Input: part model. Units: mm. Frame: model coordinates. A direction names the side the tool comes from. Give positions to 0.01 mm unless a question says otherwise; leave off trailing zeros. Loops run counter-clockwise (first coordinate to the right, second up) from the corner with the lowest first, then second, coordinate; pieces in that order, holes last. Notation, with made-up numbers: (61.5, 19.25) - (93.5, 19.25) arc R15 ccw to (93.5, 42.25) - close; hole circle Ø1 at (-32.75, 0). An arc over 180 degrees is marked (long way). Answer as a JSON object with one key per item and string values. Group by question number.
(1) Pin query (flat end, axial travel): P1, Ø8, axis at x = 6.5, y = 5.5, coming from the -Z side; P2, Ø0.8, axis at y = 13.5, z = 2.5, coming from the -X side; P3, Ø0.8, axis at x = 9.5, z = 2, coming from the -Y side; P4, Ø1.2, axis at y = 13.5, z = 2.5, coming from the +X side. Return the tip coordinate at first contact, or that it passes through.
(2) Section query D-D (z = 0.8). Count the separate pieces of the cut face and the enclosed holes in it, plus the area to 3 significant figures.
(3) Section query A-A (x = 2.5). Return loops of the section in (y, z).
(4) Material intervals for L1, parallel to X at y = 9, z = 2.1; L2, parallel to Z at x = 4.5, y = 6; L3, parallel to Y at x = 2.5, z = 0.55, sorted ascending.
(5) Access query for faces 1 (the flat face through (10, 9.7, 2)), 2 (the flat face through (8.9, 13, 2)), 3 (the flat face through (8.4, 8, 2)), 4 (the flat face through (11.9, 13, 2)). Directions: +Z, -Z, +X, -X, +Y, -Y. A direction counts if a zero-diameter tool reaches every point of the face in a straight line with its end or side. Return the directions, or none.
(6) Section query B-B (y = 13.2). Return loops of the section in (x, z), plus the area to 3 significant figures.
(7) Mould query, pull axis Y, two halves, no side actions, for faces 5 (the flat face through (3.25, 8, 2)), 6 (the flat face through (10, 14.1, 2)), 7 (the flat face through (10, 12.3, 2)). Classes: +Y half, -Y half, draft (parallel to the pull), parting line (faces both ways), or undercut.
(8) Section query C-C (z = 2.55). Return loops of the section in (x, y).
Autodesk Inventor part; units mm, degrees
ref_plane "YZ Plane" through (0, 0, 0) normal (1, 0, 0) x (0, 1, 0)
ref_plane "XZ Plane" through (0, 0, 0) normal (0, 1, 0) x (-1, 0, 0)
ref_plane "XY Plane" through (0, 0, 0) normal (0, 0, 1) x (1, 0, 0)
sketch "Skizze1" plane through (0, 0, 0) normal (0, 0, 1) x (1, 0, 0)
  line L0 (0, 0) -> (20.8, 0)
  line L1 (20.8, 0) -> (20.8, 15.7)
  line L2 (20.8, 15.7) -> (0, 15.7)
  line L3 (0, 15.7) -> (0, 0)
  circle A0 centre (2.5, 13.2) radius 1.55
  circle A1 centre (18.3, 13.2) radius 1.55
  dimension "d0" = 20.8
  dimension "d1" = 15.7
  dimension "d2" = 2.5
  dimension "d3" = 2.5
  dimension "d4" = 2.5
  dimension "d5" = 2.5
  dimension "d6" = 3.1
  dimension "d7" = 3.1
extrude "Grundkörper" add sketch "Skizze1" along normal blind 1.4
sketch "Skizze2" plane through (0, 0, 1.4) normal (0, 0, 1) x (1, 0, 0)
  line L0 (8.4, 5.7) -> (12.4, 5.7)
  line L1 (12.4, 5.7) -> (12.4, 9.7)
  line L2 (12.4, 9.7) -> (8.4, 9.7)
  line L3 (8.4, 9.7) -> (8.4, 5.7)
  line L4 (20.8, 0) -> (20.8, 15.7)
  line L5 (20.8, 15.7) -> (0, 15.7)
  line L6 (1.75, 6.2) -> (3.25, 6.2)
  line L7 (3.25, 6.2) -> (3.25, 9.2)
  line L8 (3.25, 9.2) -> (1.75, 9.2)
  line L9 (1.75, 9.2) -> (1.75, 6.2)
  line L10 (12.4, 7.7) -> (8.4, 7.7) construction
  line L11 (3.25, 7.7) -> (1.75, 7.7) construction
  line L12 (0, 15.7) -> (0, 0) construction
  line L13 (8.9, 14.1) -> (11.9, 14.1)
  line L14 (11.9, 14.1) -> (11.9, 12.3)
  line L15 (11.9, 12.3) -> (8.9, 12.3)
  line L16 (8.9, 12.3) -> (8.9, 14.1)
  line L17 (10.4, 15.7) -> (10.4, 0) construction
  line L18 (0, 0) -> (20.8, 0) construction
  line L19 (10.4, 9.7) -> (10.4, 5.7) construction
  circle A0 centre (2.5, 13.2) radius 1.55 construction
  circle A1 centre (18.3, 13.2) radius 1.55 construction
  line L20 (2.5, 13.2) -> (18.3, 13.2) construction
  line L21 (10.4, 14.1) -> (10.4, 12.3) construction
  line L22 (8.9, 13.2) -> (11.9, 13.2) construction
  line L23 (2.5, 13.2) -> (2.5, 11.65) construction
  line L24 (2.5, 9.2) -> (2.5, 6.2) construction
  dimension "d10" = 4
  dimension "d11" = 4
  dimension "d13" = 6
  dimension "d14" = 3
  dimension "d15" = 1.5
  dimension "d17" = 1.8
  dimension "d18" = 3
extrude "SMDs" add sketch "Skizze2" along normal blind 1.5
sketch "Skizze3" plane through (0, 0, 1.4) normal (0, 0, 1) x (1, 0, 0)
  line L0 (20.8, 15.7) -> (0, 15.7) construction
  line L1 (10.4, 15.7) -> (10.4, 0) construction
  line L2 (0, 0) -> (20.8, 0) construction
  line L3 (0, 15.7) -> (0, 0) construction
  line L4 (0, 1.6) -> (20.8, 1.6) construction
  line L5 (20.8, 0) -> (20.8, 15.7) construction
  point P0 (19.225, 1.6132)
  point P1 (16.685, 1.6132)
  point P2 (14.145, 1.6132)
  point P3 (11.605, 1.6132)
  point P4 (9.065, 1.6132)
  point P5 (6.525, 1.6132)
  point P6 (3.985, 1.6132)
  point P7 (1.445, 1.6132)
  dimension "d28" = 14.1
  dimension "d29" = 17.65
  dimension "d33" = 2.54
hole "Bohrung1" at (19.225, 1.6132, 1.4) at (16.685, 1.6132, 1.4) at (14.145, 1.6132, 1.4) at (11.605, 1.6132, 1.4) at (9.065, 1.6132, 1.4) at (6.525, 1.6132, 1.4) at (3.985, 1.6132, 1.4) at (1.445, 1.6132, 1.4) direction (0, 0, -1) diameter 0.75 end through all
ref_plane "Work Plane1" through (0, 0, 0.7) normal (0, 0, 1) x (1, 0, 0)
properties part number "GY_521"
Recorded:
{
 "1": {"P1": "stops at z = 0", "P2": "stops at x = 8.9", "P3": "stops at y = 5.7", "P4": "stops at x = 11.9"},
 "2": {"separate pieces": "1", "enclosed holes": "10", "area": "308 mm^2"},
 "3": {"outline": "(0, 0) - (11.65, 0) - (11.65, 1.4) - (9.2, 1.4) - (9.2, 2.9) - (6.2, 2.9) - (6.2, 1.4) - (0, 1.4) - close; (14.75, 0) - (15.7, 0) - (15.7, 1.4) - (14.75, 1.4) - close"},
 "4": {"L1": "x = 1.75 to 3.25, 8.4 to 12.4", "L2": "z = 0 to 1.4", "L3": "y = 0 to 11.65, 14.75 to 15.7"},
 "5": {"face 1": "+Z, +X, -X", "face 2": "+Z, -X, +Y", "face 3": "+Z, +Y, -Y", "face 4": "+Z, +X, +Y"},
 "6": {"outline": "(0, 0) - (0.95, 0) - (0.95, 1.4) - (0, 1.4) - close; (4.05, 0) - (16.75, 0) - (16.75, 1.4) - (11.9, 1.4) - (11.9, 2.9) - (8.9, 2.9) - (8.9, 1.4) - (4.05, 1.4) - close; (19.85, 0) - (20.8, 0) - (20.8, 1.4) - (19.85, 1.4) - close", "area": "24.9 mm^2"},
 "7": {"face 5": "draft", "face 6": "+Y half", "face 7": "undercut"},
 "8": {"outline": "(1.75, 6.2) - (3.25, 6.2) - (3.25, 9.2) - (1.75, 9.2) - close; (8.4, 5.7) - (12.4, 5.7) - (12.4, 9.7) - (8.4, 9.7) - close; (8.9, 12.3) - (11.9, 12.3) - (11.9, 14.1) - (8.9, 14.1) - close"}
}
